The figure shows three views and two pictorial views of one solid part (mm, origin at its lowest corner). Answer the questions. A direction names the side the tool comes from. Round coordinates to 2 decimals unless told otherwise and drop trailing zeros. Order: outer loops, then holes, each group sorted by start corner. A loop starts at its lowest first (then second) coordinate and runs counter-clockwise, first axis right, second up. Notation, with made-up numbers: M 20.25,70.25 L 77.25,70.25 A9 cw 77.25,76.25 Z; hole C 26,23 d3. An arc over 180 degrees is marked long. Answer as CSV lines item,"result".
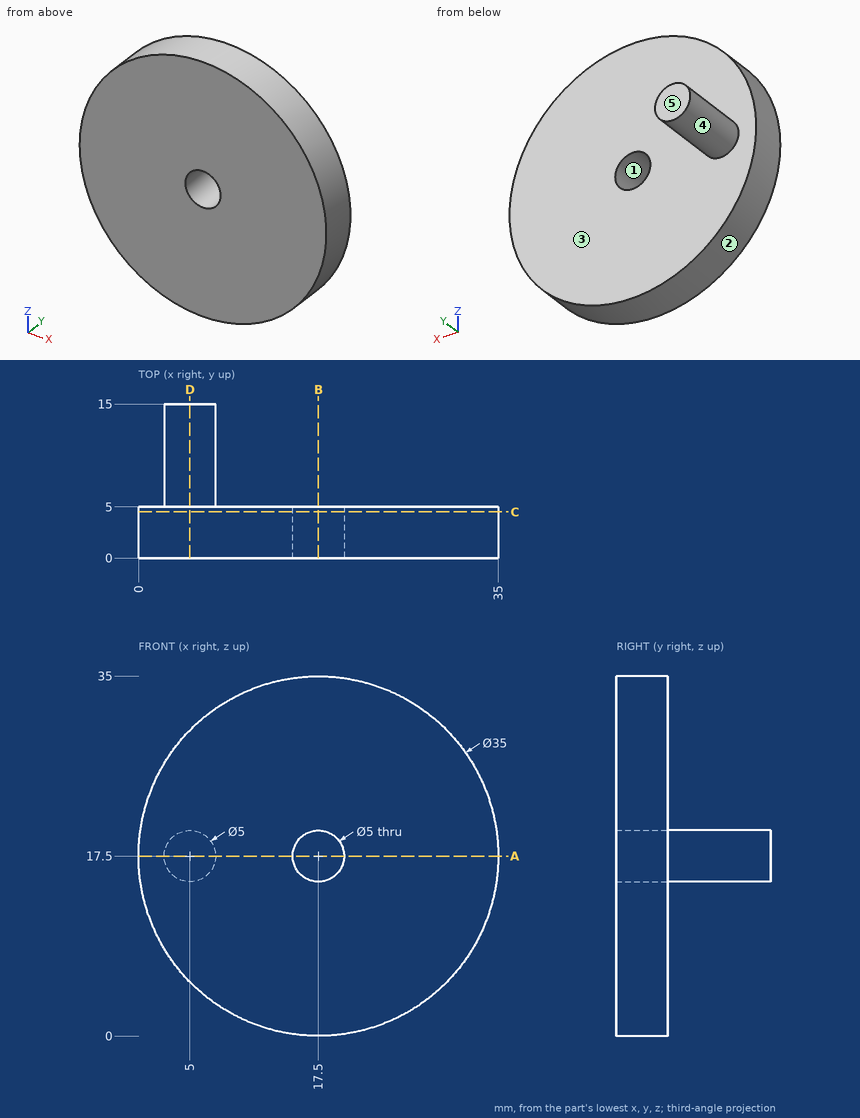
Item 1: A cutting plane is placed at A-A, the plane z = 17.5. Determine the outline of the cut face in (x, y), and give its area (3 significant figures).
Ans:
outline,"M 0,0 L 15,0 L 15,5 L 7.5,5 L 7.5,15 L 2.5,15 L 2.5,5 L 0,5 Z; M 20,0 L 35,0 L 35,5 L 20,5 Z"
area,"200 mm2"
Item 2: Determine the mould class of the marked faces 1, 2 and 3 for opening direction Z: +Z half, -Z half, draft (parallel to the pull), parting line (faces both ways), or undercut.
Ans:
face 1,"undercut"
face 2,"parting line"
face 3,"draft"
Item 3: A tool of negligible diameter and unlimited length cuts with its end or side. For the marked faces 4 and 5, from which of +Z, -Z, +X, -X, +Y, -Y can it reach the whole face along a straight path? Write none if from no direction.
Ans:
face 4,"+Y"
face 5,"+Z, -Z, +X, -X, +Y"
Item 4: A cutting plane is placed at B-B, the plane x = 17.5. Determine the outline of the cut face in (y, z).
Ans:
outline,"M 0,0 L 5,0 L 5,15 L 0,15 Z; M 0,20 L 5,20 L 5,35 L 0,35 Z"
Item 5: A cutting plane is placed at C-C, the plane y = 4.5. Determine the outline of the cut face in (x, z), and give its area (3 significant figures).
Ans:
outline,"C 17.5,17.5 d35; hole C 17.5,17.5 d5"
area,"942 mm2"
Item 6: A cutting plane is placed at D-D, the plane x = 5. Determine the outline of the cut face in (y, z).
Ans:
outline,"M 0,5.25 L 5,5.25 L 5,15 L 15,15 L 15,20 L 5,20 L 5,29.75 L 0,29.75 Z"
Item 7: Flat-ended cylindrical pins translate along their axes: pin 1 (4 mm diameter, centred on x = 6.5, z = 23.5, fed in from +Y); pin 2 (1 mm diameter, centred on x = 5.5, y = 13.5, fed in from +Z); pin 3 (3 mm diameter, centred on x = 31, y = 4, fed in from -Z). Find the tip coordinate at first contact, or state that the pin passes through.
Ans:
pin 1,"y = 5"
pin 2,"z = 20"
pin 3,"z = 4.76"
Item 8: Find the intervals of material crossed by probe 1 along Z at (x, y) = (17.5, 3); probe 2 along Y at (x, z) = (17, 8.5); probe 3 along Z at (x, y) = (3, 6), in increasing order. Write a range as [from, to].
Ans:
probe 1,"[0, 15], [20, 35]"
probe 2,"[0, 5]"
probe 3,"[16, 19]"
